from build123d import *

# Parameters (mm, degrees)
F0_W     = 38
F0_H     = 38
F1_DEPTH = 36.5
F2_R     = 5
F3_W     = 21
F3_H     = 23
F4_DEPTH = 18.5


with BuildPart() as f1:
    # F0 (on Top) → F1 (new body)
    with BuildSketch(Plane.XY):
        Rectangle(F0_W, F0_H)
    extrude(amount=F1_DEPTH)

    # F2
    f2_edges = [f1.edges().sort_by_distance(p)[0] for p in [
        (19, -19, 18.25),
        (19, 19, 18.25),
        (-19, 19, 18.25),
        (-19, -19, 18.25),
    ]]
    fillet(f2_edges, radius=F2_R)

    # F3 (on face) → F4 (join)
    with BuildSketch(Plane.XZ.offset(19)):
        with Locations((0, 16)):
            Rectangle(F3_W, F3_H)
    extrude(amount=F4_DEPTH)


solid = f1.part
Here's how the part is built. I have some questions about the finished solid (model axes, mm). A direction names the side the tool comes from. Coordinates: 2 decimals unless noted, no trailing zeros. Loops run counter-clockwise (first coordinate to the right, second up) from the corner with the lowest first, then second, coordinate; pieces in that order, holes last.
1. For P1, Ø6, axis at x = 9, z = 32.5, coming from the -Y side; P2, Ø15, axis at x = -1.5, y = -32, coming from the -Z side; P3, Ø15, axis at y = -33, z = 14.5, coming from the +X side, each with a flat end and sliding along its axis, tell me the tip position at first contact or that it passes through.
2. I need wall thicknesses on L1, parallel to X at y = -30.5, z = 25; L2, parallel to Y at x = -5, z = 32.5; L3, parallel to Z at x = 2.5, y = -29.5. Which ranges of each line are inside material? Lowest first, please.
3. Imagine slicing it at C-C, the plane y = -32. Please give me the cut outline in (x, z), and give its area (3 significant figures).
4. For faces 1 (the flat face through (0, -28, 4.5)), 2 (the flat face through (0, -28, 27.5)), 3 (the flat face through (-10.5, -28, 16)), which set-ups out of +Z, -Z, +X, -X, +Y, -Y let a thin tool reach every point of the face, with its end or its side?
5. Imagine slicing it at A-A, the plane x = 8.5. Please give me the cut outline in (y, z).
6. Imagine slicing it at D-D, the plane z = 31. Please give me the cut outline in (x, y).
7. Imagine slicing it at B-B, the plane z = 12. Please give me the cut outline in (x, y), and give its area (3 significant figures).
Taken from the geometry:
1. P1: stops at y = -19
1. P2: stops at z = 4.5
1. P3: stops at x = 10.5
2. L1: x = -10.5 to 10.5
2. L2: y = -19 to 19
2. L3: z = 4.5 to 27.5
3. outline: (-10.5, 4.5) - (10.5, 4.5) - (10.5, 27.5) - (-10.5, 27.5) - close
3. area: 483 mm2
4. face 1: -Z, +X, -X, -Y
4. face 2: +Z, +X, -X, -Y
4. face 3: +Z, -Z, -X, -Y
5. outline: (-37.5, 4.5) - (-19, 4.5) - (-19, 0) - (19, 0) - (19, 36.5) - (-19, 36.5) - (-19, 27.5) - (-37.5, 27.5) - close
6. outline: (-19, -14) arc R5 ccw to (-14, -19) - (14, -19) arc R5 ccw to (19, -14) - (19, 14) arc R5 ccw to (14, 19) - (-14, 19) arc R5 ccw to (-19, 14) - close
7. outline: (-19, -14) arc R5 ccw to (-14, -19) - (-10.5, -19) - (-10.5, -37.5) - (10.5, -37.5) - (10.5, -19) - (14, -19) arc R5 ccw to (19, -14) - (19, 14) arc R5 ccw to (14, 19) - (-14, 19) arc R5 ccw to (-19, 14) - close
7. area: 1,810 mm2
